```python
from build123d import *

# Parameters (mm, degrees)
F0_R     = 60
F1_DEPTH = 5
F2_R     = 1
F3_R     = 7.0850530083
F4_DEPTH = 2
F6_R     = 33.800823702
F7_DEPTH = 5
F8_SIZE2 = 4
F8_SIZE  = 12


# Not quite as in the source:
# - a fillet or chamfer that OpenCascade refuses, or shapes differently, is made with other operations: its cross-section is extruded or revolved along the edge and cut away or added
# - a feature names something its author has since deleted; it is built from what else it names


with BuildPart() as f1:
    # F0 (on Top) → F1 (new body)
    with BuildSketch(Plane.XY):
        Circle(F0_R)
    extrude(amount=F1_DEPTH)

    # F2
    f2_edges = [f1.edges().sort_by_distance(p)[0] for p in [
        (-60, 0, 5),
    ]]
    fillet(f2_edges, radius=F2_R)

    # F3 (on face) → F4 (join)
    with BuildSketch(Plane.XY.offset(5)):
        with Locations((0, 47)):
            Circle(F3_R)
        with Locations((-44.6996562659, 14.5237987356)):
            Circle(F3_R)
        with Locations((-27.6259068577, -38.0237987356)):
            Circle(F3_R)
        with Locations((27.6259068577, -38.0237987356)):
            Circle(F3_R)
        with Locations((44.6996562659, 14.5237987356)):
            Circle(F3_R)
    extrude(amount=F4_DEPTH)

    # F5: fillet of radius 5 on 5 edges, made by hand

    # F5_s1 → F5_t2 (revolve, cut)
    with BuildSketch(Plane.XZ.offset(-47)):
        with BuildLine():
            ThreePointArc((7.0850530083, 5), (5.3211209858, 6.472135955), (3.0850530083, 7))
            Line((3.0850530083, 7), (7.0850530083, 7))
            Line((7.0850530083, 7), (7.0850530083, 5))
        make_face()
    revolve(axis=Axis((0, 47, 7), (0, 0, 1)), mode=Mode.SUBTRACT)

    # F5_s3 → F5_t4 (revolve, cut)
    with BuildSketch(Plane.XZ.offset(-14.5237987356)):
        with BuildLine():
            ThreePointArc((51.7847092742, 5), (50.0207772517, 6.472135955), (47.7847092742, 7))
            Line((47.7847092742, 7), (51.7847092742, 7))
            Line((51.7847092742, 7), (51.7847092742, 5))
        make_face()
    revolve(axis=Axis((44.6996562659, 14.5237987356, 7), (0, 0, 1)), mode=Mode.SUBTRACT)

    # F5_s5 → F5_t6 (revolve, cut)
    with BuildSketch(Plane.XZ.offset(38.0237987356)):
        with BuildLine():
            ThreePointArc((34.7109598661, 5), (32.9470278436, 6.472135955), (30.7109598661, 7))
            Line((30.7109598661, 7), (34.7109598661, 7))
            Line((34.7109598661, 7), (34.7109598661, 5))
        make_face()
    revolve(axis=Axis((27.6259068577, -38.0237987356, 7), (0, 0, 1)), mode=Mode.SUBTRACT)

    # F5_s7 → F5_t8 (revolve, cut)
    with BuildSketch(Plane.XZ.offset(38.0237987356)):
        with BuildLine():
            ThreePointArc((-20.5408538494, 5), (-22.3047858719, 6.472135955), (-24.5408538494, 7))
            Line((-24.5408538494, 7), (-20.5408538494, 7))
            Line((-20.5408538494, 7), (-20.5408538494, 5))
        make_face()
    revolve(axis=Axis((-27.6259068577, -38.0237987356, 7), (0, 0, 1)), mode=Mode.SUBTRACT)

    # F5_s9 → F5_t10 (revolve, cut)
    with BuildSketch(Plane.XZ.offset(-14.5237987356)):
        with BuildLine():
            ThreePointArc((-37.6146032575, 5), (-39.37853528, 6.472135955), (-41.6146032575, 7))
            Line((-41.6146032575, 7), (-37.6146032575, 7))
            Line((-37.6146032575, 7), (-37.6146032575, 5))
        make_face()
    revolve(axis=Axis((-44.6996562659, 14.5237987356, 7), (0, 0, 1)), mode=Mode.SUBTRACT)

    # F6 (on face) → F7 (join)
    with BuildSketch(Plane.XY.offset(5)):
        Circle(F6_R)
    extrude(amount=F7_DEPTH)

    # F8
    f8_edges = [f1.edges().sort_by_distance(p)[0] for p in [
        (-33.800824, 0, 10),
    ]]
    f8_side = f1.faces().sort_by_distance((0, 0, 10))[0]
    chamfer(f8_edges, length=F8_SIZE, length2=F8_SIZE2, reference=f8_side)

    # F9: fillet of radius 2 on 1 edges, made by hand

    # F9_s1 → F9_t2 (revolve, cut)
    with BuildSketch(Plane.XZ):
        with BuildLine():
            ThreePointArc((33.800823702, 5), (33.33069476, 5.8898153625), (32.486741959, 6.4380272477))
            Line((32.486741959, 6.4380272477), (33.800823702, 6))
            Line((33.800823702, 6), (33.800823702, 5))
        make_face()
    revolve(axis=Axis((0, 0, 6), (0, 0, 1)), mode=Mode.SUBTRACT)


solid = f1.part
```
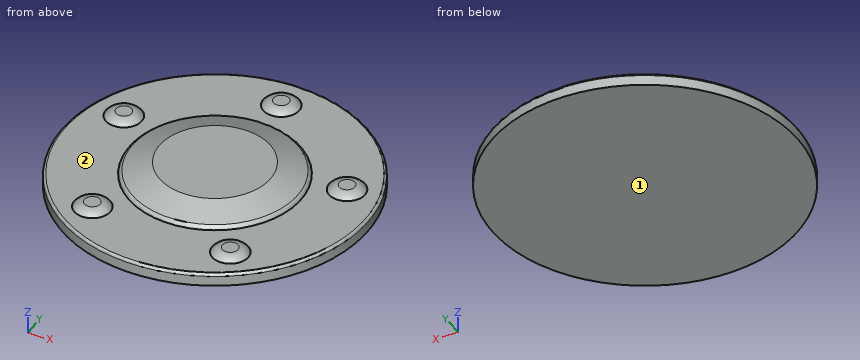
The model under review builds one solid part; all positions refer to its coordinate system, in mm. Face numbers are marked on the shaded views. A direction names the side the tool comes from. Coordinates: 2 decimals unless noted, no trailing zeros. Write each loop counter-clockwise with the first axis right and the second up, starting at its lowest first coordinate (ties: lowest second). Pieces come first, ordered by that corner, then holes.
1) We need section A-A on y = 0. State the section outline as (x, z) points.
2) Machinability: for the marked faces 1 and 2, which of the approach directions +Z, -Z, +X, -X, +Y, -Y give a long, thin tool a straight path to every point of the face, cutting with its end or side? Answer none if there is none.
3) We need section B-B on z = 8.5. State the section outline as (x, y) points, then the cut area to 3 significant figures.
4) To check wall thickness, follow probe 1 along Z at (x, y) = (29, -21); probe 2 along Z at (x, y) = (29, -37.5); probe 3 along Y at (x, z) = (18, 1.5). State the ranges of each line that lie inside material, in increasing order.
5) Clearance check with flat-ended pins moving along their axes: pin 1 Ø1.9 at (x, y) = (-29, -37.5) entering from +Z; pin 2 Ø6 at (y, z) = (-35.5, 4.5) entering from -X; pin 3 Ø4 at (x, z) = (47.5, 8) entering from +Y. State where each tip first meets the part, or that it passes through.
Answer list:
1. outline: (-60, 0) - (60, 0) - (60, 4) arc R1 ccw to (59, 5) - (33.8, 5) arc R2 ccw to (32.49, 6.44) - (21.8, 10) - (-21.8, 10) - (-32.49, 6.44) arc R2 ccw to (-33.8, 5) - (-59, 5) arc R1 ccw to (-60, 4) - close
2. face 1: -Z, +X, -X, +Y, -Y
2. face 2: +Z
3. outline: circle Ø52.6 at (0, 0)
3. area: 2,170 mm2
4. probe 1: z = 0 to 5
4. probe 2: z = 0 to 7
4. probe 3: y = -57.24 to 57.24
5. pin 1: stops at z = 7
5. pin 2: stops at x = -50.41
5. pin 3: stops at y = 20.06
